Can you work these out from the model? Positions are in its coordinate system, mm. A direction names the side the tool comes from. Coordinates: 2 decimals unless noted, no trailing zeros. Loops run counter-clockwise (first coordinate to the right, second up) from the corner with the lowest first, then second, coordinate; pieces in that order, holes last.
```python
from build123d import *

# Parameters (mm, degrees)
SKETCH1_W          = 50.8
SKETCH1_H          = 50.8
MAIN_BODY_DEPTH    = 18.288
SKETCH2_W          = 7.112
SKETCH2_H          = 28.448
FRONT_CUT_DEPTH    = 75.133197314
SHELL1_T           = -2.032
SKETCH3_R          = 13.5001
CENTER_HOLE_DEPTH  = 75.133197314
FILL060_VERT_R     = 1.524
FILL060_TB_R       = 1.524
CHAM025_SIZE       = 0.635
KEYED_HOLE_1_DEPTH = 58.653742931


with BuildPart() as part:
    # Sketch1 → main body (new body)
    with BuildSketch(Plane.XY):
        with Locations((25.4, 25.4)):
            Rectangle(SKETCH1_W, SKETCH1_H)
    extrude(amount=MAIN_BODY_DEPTH)

    # Sketch2 → front cut (cut, through all)
    with BuildSketch(Plane(origin=(50.8, 0, 0), x_dir=(0, 0, -1), z_dir=(1, 0, 0))):
        with Locations((-14.732, 36.576)):
            Rectangle(SKETCH2_W, SKETCH2_H)
    extrude(amount=-FRONT_CUT_DEPTH, mode=Mode.SUBTRACT)

    # Shell1
    shell1_openings = [part.faces().sort_by_distance(p)[0] for p in [
        (25.4, 36.576, 11.176),
        (25.4, 22.352, 14.732),
    ]]
    offset(amount=SHELL1_T, openings=shell1_openings, kind=Kind.INTERSECTION)

    # Sketch3 → center hole (cut, through all)
    with BuildSketch(Plane.XY):
        with Locations((25.4, 22.352)):
            Circle(SKETCH3_R)
    extrude(amount=CENTER_HOLE_DEPTH, mode=Mode.SUBTRACT)

    # fill060.vert
    fill060_vert_edges = [part.edges().sort_by_distance(p)[0] for p in [
        (2.032, 12.192, 16.256),
        (48.768, 12.192, 16.256),
        (2.032, 25.4, 2.032),
        (48.768, 25.4, 2.032),
    ]]
    fillet(fill060_vert_edges, radius=FILL060_VERT_R)

    # fill060.tb
    fill060_tb_edges = [part.edges().sort_by_distance(p)[0] for p in [
        (2.032, 48.768, 7.366),
        (48.768, 48.768, 7.366),
        (25.4, 2.032, 16.256),
        (25.4, 2.032, 2.032),
        (2.032, 2.032, 9.144),
        (48.768, 2.032, 9.144),
        (2.478369265, 2.032, 15.809630735),
        (2.478369265, 2.032, 2.478369265),
        (48.321630735, 2.032, 2.478369265),
        (48.321630735, 2.032, 15.809630735),
        (25.4, 48.768, 2.032),
        (2.478369265, 48.768, 2.478369265),
        (48.321630735, 48.768, 2.478369265),
    ]]
    fillet(fill060_tb_edges, radius=FILL060_TB_R)

    # cham025
    cham025_edges = [part.edges().sort_by_distance(p)[0] for p in [
        (11.8999, 22.352, 0),
        (25.4, 8.8519, 18.288),
    ]]
    chamfer(cham025_edges, length=CHAM025_SIZE)

    # Sketch6 → Keyed Hole 1 (cut, through all)
    with BuildSketch(Plane(origin=(13.426773448, 39.909210303, 0), x_dir=(0, 1, 0), z_dir=(0, 0, -1))):
        with BuildLine():
            Line((1.238789697, 0.162226552), (2.635789697, 0.162226552))
            Line((2.635789697, 0.162226552), (2.635789697, -1.615773448))
            Line((2.635789697, -1.615773448), (1.238789697, -1.615773448))
            ThreePointArc((1.238789697, -1.615773448), (-4.984210303, -0.726773448), (1.238789697, 0.162226552))
        make_face()
    extrude(amount=-KEYED_HOLE_1_DEPTH, mode=Mode.SUBTRACT)


solid = part.part
```
(1) I want a section at D-D on y = 5. Write out the boundary of the cut face in (x, z).
Check values:
outline: (0, 0) - (50.8, 0) - (50.8, 18.29) - (0, 18.29) - close; hole (2.03, 3.56) arc R1.52 ccw to (3.56, 2.03) - (47.24, 2.03) arc R1.52 ccw to (48.77, 3.56) - (48.77, 14.73) arc R1.52 ccw to (47.24, 16.26) - (3.56, 16.26) arc R1.52 ccw to (2.03, 14.73) - close
(2) I want a section at A-A on x = 25.4. Write out the boundary of the cut face in (y, z) (3 decimals).
Check values:
outline: (0, 0) - (8.217, 0) - (8.852, 0.635) - (8.852, 2.032) - (3.556, 2.032) arc R1.524 cw to (2.032, 3.556) - (2.032, 14.732) arc R1.524 cw to (3.556, 16.256) - (8.852, 16.256) - (8.852, 17.653) - (8.217, 18.288) - (0, 18.288) - close; (35.852, 0.635) - (36.487, 0) - (50.8, 0) - (50.8, 11.176) - (48.768, 11.176) - (48.768, 3.556) arc R1.524 cw to (47.244, 2.032) - (35.852, 2.032) - close
(3) I want a section at C-C on z = 9.75. Write out the boundary of the cut face in (x, y), then the cut area to 3 significant figures.
Check values:
outline: (0, 0) - (50.8, 0) - (50.8, 50.8) - (0, 50.8) - close; hole (2.03, 3.56) arc R1.52 ccw to (3.56, 2.03) - (47.24, 2.03) arc R1.52 ccw to (48.77, 3.56) - (48.77, 47.24) arc R1.52 ccw to (47.24, 48.77) - (3.56, 48.77) arc R1.52 ccw to (2.03, 47.24) - close
area: 398 mm2
(4) I want a section at B-B on y = 38.1. Write out the boundary of the cut face in (x, z) (3 decimals), then the cut area to 3 significant figures.
Check values:
outline: (0, 0) - (9.525, 0) - (9.525, 2.032) - (3.556, 2.032) arc R1.524 cw to (2.032, 3.556) - (2.032, 11.176) - (0, 11.176) - close; (15.875, 0) - (50.8, 0) - (50.8, 11.176) - (48.768, 11.176) - (48.768, 3.556) arc R1.524 cw to (47.244, 2.032) - (15.875, 2.032) - close
area: 128 mm2
(5) I'm going to push a flat-ended pin straight in: pin 1 (2 mm diameter, centred on x = 45.5, z = 15.5, fed in from +Y). Where does the tip first touch, or does it pass through?
Check values:
pin 1: stops at y = 22.35
(6) Which directions (+Z, -Z, +X, -X, +Y, -Y) give clear straight access to the entire face, cutting with the end or side of a thin tool? Please do faces 4 (the cylindrical face through (2.467, 48.31, 7.313)), 5 (the cylindrical face through (12.573, 34.928, 1.002)), 6 (the flat face through (2.032, 25, 8)).
Check values:
face 4: +Z
face 5: +Z, -Z
face 6: none
(7) If I drill on probe 1 along X at (y, z) = (38.1, 1.65) (3 decimals); probe 2 along Y at (x, z) = (25.4, 1.55); probe 3 along Y at (x, z) = (4, 5.5), over which ranges is the centre line in solid material (lowest first)?
Check values:
probe 1: x = 0 to 9.525, 15.875 to 50.8
probe 2: y = 0 to 8.85, 35.85 to 50.8
probe 3: y = 0 to 2.03, 48.77 to 50.8
(8) If we mould it in two halves opening along Y, with no side actions, what happens to faces 1 (the flat face through (25, 6, 18.288)), 2 (the flat face through (13, 42.545, 1)), 3 (the flat face through (25, 50.8, 6))? For each: released by +Y, released by -Y, zero draft, split by the parting line, or undercut.
Check values:
face 1: zero draft
face 2: undercut
face 3: released by +Y
